Could you check a few things on this drawing? It's one solid part, dimensions in mm from its lowest x, y, z. A direction names the side the tool comes from. Coordinates: 2 decimals unless noted, no trailing zeros. Write each loop counter-clockwise with the first axis right and the second up, starting at its lowest first coordinate (ties: lowest second). Pieces come first, ordered by that corner, then holes. Notation, with made-up numbers: M 7,14.5 L 42,14.5 A23 cw 42,24.5 Z; hole C 37,25.25 d8. An arc over 180 degrees is marked long. Use a Markdown table: item, result.
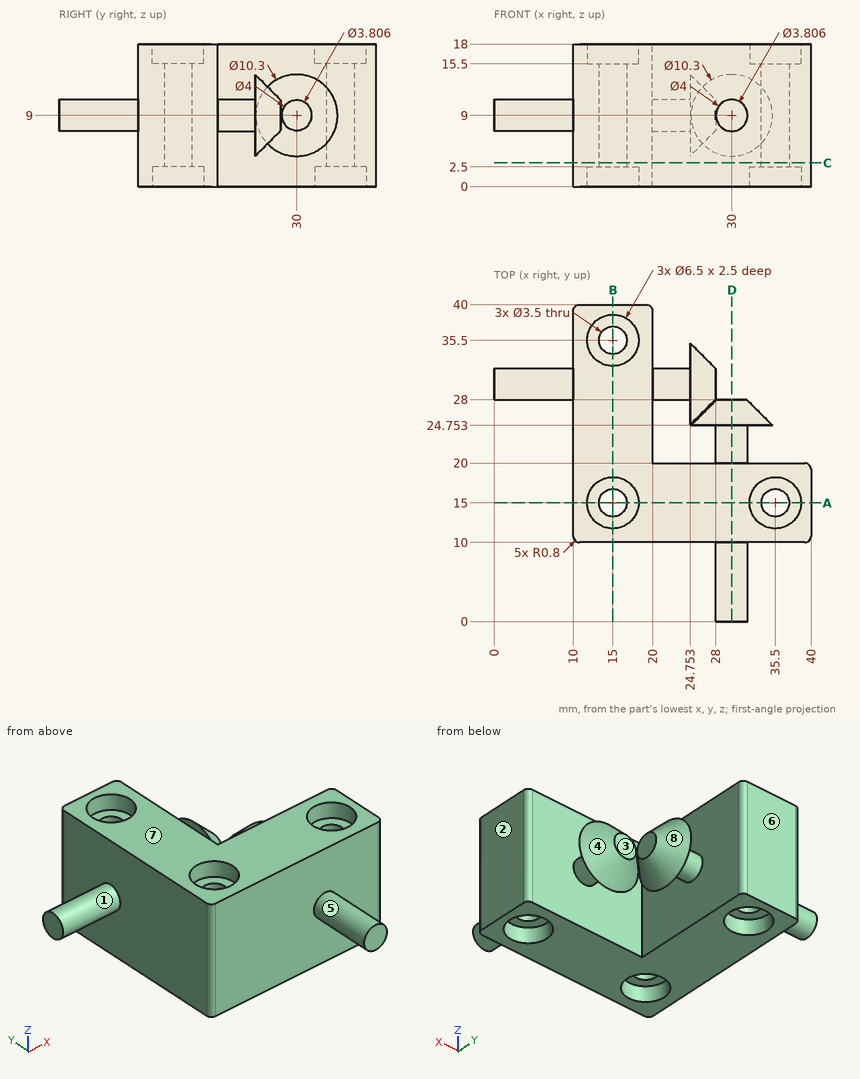
1. Suppose I cut it at A-A on y = 15. Write out the boundary of the cut face in (x, z).
Answers follow:
| item | result |
|---|---|
| outline | M 10,0 L 11.75,0 L 11.75,2.5 L 13.25,2.5 L 13.25,15.5 L 11.75,15.5 L 11.75,18 L 10,18 Z; M 16.75,2.5 L 18.25,2.5 L 18.25,0 L 32.25,0 L 32.25,2.5 L 33.75,2.5 L 33.75,15.5 L 32.25,15.5 L 32.25,18 L 18.25,18 L 18.25,15.5 L 16.75,15.5 Z; M 37.25,2.5 L 38.75,2.5 L 38.75,0 L 40,0 L 40,18 L 38.75,18 L 38.75,15.5 L 37.25,15.5 Z |
2. Which directions (+Z, -Z, +X, -X, +Y, -Y) give clear straight access to the entire face, cutting with the end or side of a thin tool? Please do the marked faces 1, 2, 3, 4 and 5.
Answers follow:
| item | result |
|---|---|
| face 1 | -X |
| face 2 | +Z, -Z, +X, +Y, -Y |
| face 3 | +Z, -Z, +X, +Y |
| face 4 | none |
| face 5 | -Y |
3. I need wall thicknesses on probe 1 along Y at (x, z) = (35.5, 1); probe 2 along Y at (x, z) = (35.5, 13); probe 3 along X at (y, z) = (33, 4.75). Which ranges of each line are inside material? Lowest first, please.
Answers follow:
| item | result |
|---|---|
| probe 1 | y = 10 to 11.75, 18.25 to 20 |
| probe 2 | y = 10 to 13.25, 16.75 to 20 |
| probe 3 | x = 10 to 20 |
4. Will these pins go through, and if not, where does the flat tip stop? pin 1 Ø10 at (x, z) = (22.5, 10.5) entering from -Y; pin 2 Ø2 at (x, y) = (36.5, 14) entering from -Z; pin 3 Ø7.5 at (x, y) = (15, 35.5) entering from -Z; pin 4 Ø6 at (y, z) = (28.5, 15.5) entering from +X.
Answers follow:
| item | result |
|---|---|
| pin 1 | stops at y = 10 |
| pin 2 | stops at z = 2.5 |
| pin 3 | stops at z = 0 |
| pin 4 | stops at x = 26.23 |
5. Suppose I cut it at C-C on z = 3. Write out the boundary of the cut face in (x, y).
Answers follow:
| item | result |
|---|---|
| outline | M 10,10.8 A0.8 ccw 10.8,10 L 39.2,10 A0.8 ccw 40,10.8 L 40,19.2 A0.8 ccw 39.2,20 L 20,20 L 20,39.2 A0.8 ccw 19.2,40 L 10.8,40 A0.8 ccw 10,39.2 Z; hole C 15,15 d3.5; hole C 15,35.5 d3.5; hole C 35.5,15 d3.5 |
6. Suppose I cut it at D-D on x = 30. Write out the boundary of the cut face in (y, z), and give its area (3 significant figures).
Answers follow:
| item | result |
|---|---|
| outline | M 0,7 L 10,7 L 10,0 L 20,0 L 20,7 L 24.75,7 L 24.75,3.85 L 28,7.1 L 28,10.9 L 24.75,14.15 L 24.75,11 L 20,11 L 20,18 L 10,18 L 10,11 L 0,11 Z |
| area | 262 mm2 |
7. We'd pull the mould along Y, two halves only. Please class the marked faces 6, 7 and 8: +Y half, -Y half, draft (parallel to the pull), parting line (faces both ways), or undercut.
Answers follow:
| item | result |
|---|---|
| face 6 | +Y half |
| face 7 | draft |
| face 8 | undercut |
